```python
from build123d import *

# Parameters (mm, degrees)
SKETCH_1_W          = 380
SKETCH_1_H          = 300
EXTRUDE_1_DEPTH     = 30
SKETCH_2_W          = 350
SKETCH_2_H          = 270
CUT_EXTRUDE_1_DEPTH = 0.5
FILLET_1_R          = 10


with BuildPart() as part:
    # 草图1 → 凸台-拉伸1 (new body)
    with BuildSketch(Plane.XY):
        with Locations((190, 150)):
            Rectangle(SKETCH_1_W, SKETCH_1_H)
    extrude(amount=EXTRUDE_1_DEPTH)

    # 草图2 → 切除-拉伸1 (cut)
    with BuildSketch(Plane.XY.offset(30)):
        with Locations((190, 150)):
            Rectangle(SKETCH_2_W, SKETCH_2_H)
    extrude(amount=-CUT_EXTRUDE_1_DEPTH, mode=Mode.SUBTRACT)

    # 圆角1
    fillet_1_edges = [part.edges().sort_by_distance(p)[0] for p in [
        (0, 300, 15),
        (380, 300, 15),
        (380, 0, 15),
        (0, 0, 15),
    ]]
    fillet(fillet_1_edges, radius=FILLET_1_R)


solid = part.part
```
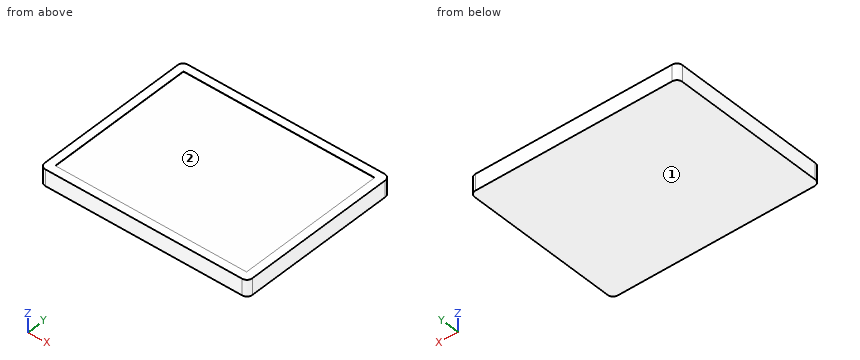
The listing builds one solid part. Answer for the finished solid, in the listing's coordinates (mm). Face numbers are marked on the shaded views. Give positions to 0.01 mm unless a question says otherwise; leave off trailing zeros. Order: outer loops, then holes, each group sorted by start corner. A loop starts at its lowest first (then second) coordinate and runs counter-clockwise, first axis right, second up. Notation, with made-up numbers: (44.25, 62.5) -> (83.25, 62.5) arc R26 ccw to (83.25, 86.5) -> close; hole circle Ø9 at (58.25, 64). An arc over 180 degrees is marked (long way). Write each question's results on one line, items separated by ' | '.
Q1. Determine the mould class of the marked faces 1 and 2 for opening direction X: pulls with the +X half, pulls with the -X half, needs draft (parallel to the pull), parting line crosses it, or undercut.
Checked values:
face 1: needs draft | face 2: undercut
Q2. This flat-tipped pin is pushed along its axis until it touches: P1, Ø1, axis at x = 157.5, y = 70, coming from the +Z side. Where does it stop, or does it pass through?
Checked values:
P1: stops at z = 29.5
Q3. The part is cut by section B-B, the plane x = 103. Give the vertices of the cut face in (y, z).
Checked values:
outline: (0, 0) -> (300, 0) -> (300, 30) -> (285, 30) -> (285, 29.5) -> (15, 29.5) -> (15, 30) -> (0, 30) -> close
Q4. A straight line is drawn through the part: probe 1 along Z at (x, y) = (51.5, 61). Find the intervals that lie inside material, in ascending order. Write a range as from..to.
Checked values:
probe 1: z = 0..29.5
Q5. The part is cut by section A-A, the plane y = 244. Give the vertices of the cut face in (x, z).
Checked values:
outline: (0, 0) -> (380, 0) -> (380, 30) -> (365, 30) -> (365, 29.5) -> (15, 29.5) -> (15, 30) -> (0, 30) -> close
